from build123d import *

# Parameters (mm, degrees)
PAD_DEPTH         = 0.25
PAD001_DEPTH      = 2.54
PAD001_DEPTH_BACK = 1.02


with BuildPart() as pad:
    # Sketch → Pad (new body, symmetric)
    with BuildSketch(Plane.XZ):
        Polygon((-1.2, 2), (-1.2, 0), (-0.635, 0), (-0.635, -16), (0, -17), (0.635, -16), (0.635, 0), (1.2, 0), (1.2, 2), align=None)
        Polygon((14.605, 0), (14.605, -16), (15.24, -17), (15.875, -16), (15.875, 0), (16.44, 0), (16.44, 2), (14.04, 2), (14.04, 0), align=None)
        Polygon((3.88, 2), (3.88, 0), (4.445, 0), (4.445, -16), (5.08, -17), (5.715, -16), (5.715, 0), (6.28, 0), (6.28, 2), align=None)
        Polygon((8.96, 2), (8.96, -0.056881), (9.525, -0.056881), (9.525, -16), (10.16, -17), (10.795, -16), (10.795, -0.056881), (11.36, -0.056881), (11.36, 2), align=None)
    extrude(amount=PAD_DEPTH, both=True)


with BuildPart() as obj1:
    # Sketch001 → Pad001 (new body, two sides)
    with BuildSketch(Plane(origin=(15.24, 0, 0), x_dir=(-1, 0, 0), z_dir=(0, 1, 0))) as pad001_sk:
        with BuildLine():
            Line((-2.78, 1.9), (18.02, 1.9))
            ThreePointArc((18.02, 1.9), (18.055355, 1.914645), (18.07, 1.95))
            Line((18.07, 1.95), (18.07, 9.43))
            Line((18.07, 9.43), (14.9, 12.6))
            Line((14.9, 12.6), (-2.78, 12.6))
            ThreePointArc((-2.78, 12.6), (-2.815355, 12.585355), (-2.83, 12.55))
            Line((-2.83, 12.55), (-2.83, 1.95))
            ThreePointArc((-2.83, 1.95), (-2.815355, 1.914645), (-2.78, 1.9))
        make_face()
    extrude(amount=PAD001_DEPTH)
    extrude(pad001_sk.sketch, amount=-PAD001_DEPTH_BACK)

    add(pad.part)


solid = obj1.part
Design review of the part built by this model. Coordinates are the model's own, in mm. A direction names the side the tool comes from. Round coordinates to 2 decimals unless told otherwise and drop trailing zeros. Loops run counter-clockwise (first coordinate to the right, second up) from the corner with the lowest first, then second, coordinate; pieces in that order, holes last. Notation, with made-up numbers: (26.5, -23) -> (71.5, -23) arc R9 ccw to (71.5, -18) -> close; hole circle Ø11 at (71.5, -20). An arc over 180 degrees is marked (long way). Use one line per item in the form item = value. Start each with the question number.
Q1. Machinability: for faces 1 (the face through (10, -0.25, -7)), 2 (the face through (-2.83, 1, 6)), 3 (the face through (10, 0.25, -7)), which of the approach directions +Z, -Z, +X, -X, +Y, -Y give a long, thin tool a straight path to every point of the face, cutting with its end or side? Answer none if there is none.
Q2. We need section A-A on z = 1.25. Give the boundary of the cut face in (x, y).
Q3. Wall thickness on line 1 along X through (y, z) = (-0.1, 0.25); line 2 along Z through (x, y) = (9.75, -0.65); line 3 along Y through (x, z) = (4.75, -13): over which ranges is each line inside the solid? List them lowest first. Write a range as [from, to].
Q4. For pin 1 Ø0.6 at (x, y) = (11, 0) entering from -Z; pin 2 Ø2.5 at (x, z) = (10.5, -4) entering from +Y; pin 3 Ø0.6 at (y, z) = (0, -10) entering from +X (3 decimals), all flat-tipped, find the tip position at first contact; note any pin that passes through.
Q5. We need section D-D on x = 10.5. Give the boundary of the cut face in (y, z).
Q6. We need section B-B on y = 0.9. Give the boundary of the cut face in (x, z), then the cut area to 3 significant figures.
Q7. We need section C-C on z = -7. Give the boundary of the cut face in (x, y) (3 decimals), then the cut area to 3 significant figures.
Calculated:
q1.face_1 = -Z, +X, -X, -Y
q1.face_2 = +Z, -Z, -X, +Y, -Y
q1.face_3 = -Z, +X, -X, +Y
q2.outline = (-1.2, -0.25) -> (1.2, -0.25) -> (1.2, 0.25) -> (-1.2, 0.25) -> close; (3.88, -0.25) -> (6.28, -0.25) -> (6.28, 0.25) -> (3.88, 0.25) -> close; (8.96, -0.25) -> (11.36, -0.25) -> (11.36, 0.25) -> (8.96, 0.25) -> close; (14.04, -0.25) -> (16.44, -0.25) -> (16.44, 0.25) -> (14.04, 0.25) -> close
q3.line_1 = [-1.2, 1.2], [3.88, 6.28], [8.96, 11.36], [14.04, 16.44]
q3.line_2 = [1.9, 12.6]
q3.line_3 = [-0.25, 0.25]
q4.pin_1 = -16.15
q4.pin_2 = 0.25
q4.pin_3 = 15.875
q5.outline = (-1.02, 1.9) -> (-0.25, 1.9) -> (-0.25, -16.46) -> (0.25, -16.46) -> (0.25, 1.9) -> (2.54, 1.9) -> (2.54, 12.6) -> (-1.02, 12.6) -> close
q6.outline = (-2.83, 1.95) arc R0.05 ccw to (-2.78, 1.9) -> (18.02, 1.9) arc R0.05 ccw to (18.07, 1.95) -> (18.07, 12.55) arc R0.05 ccw to (18.02, 12.6) -> (0.34, 12.6) -> (-2.83, 9.43) -> close
q6.area = 219 mm²
q7.outline = (-0.635, -0.25) -> (0.635, -0.25) -> (0.635, 0.25) -> (-0.635, 0.25) -> close; (4.445, -0.25) -> (5.715, -0.25) -> (5.715, 0.25) -> (4.445, 0.25) -> close; (9.525, -0.25) -> (10.795, -0.25) -> (10.795, 0.25) -> (9.525, 0.25) -> close; (14.605, -0.25) -> (15.875, -0.25) -> (15.875, 0.25) -> (14.605, 0.25) -> close
q7.area = 2.54 mm²
